Input: dimensioned drawing with shaded views. Units: mm. Origin: part minimum x, y, z. Round coordinates to 2 decimals unless told otherwise and drop trailing zeros. Loops run counter-clockwise (first coordinate to the right, second up) from the corner with the lowest first, then second, coordinate; pieces in that order, holes last. Notation, with made-up numbers: M -1,84 L 38,84 A17 ccw 38,95 Z; hole C 56,4.25 d2. An arc over 180 degrees is marked long. Return JSON: item names as keys, results as strings.
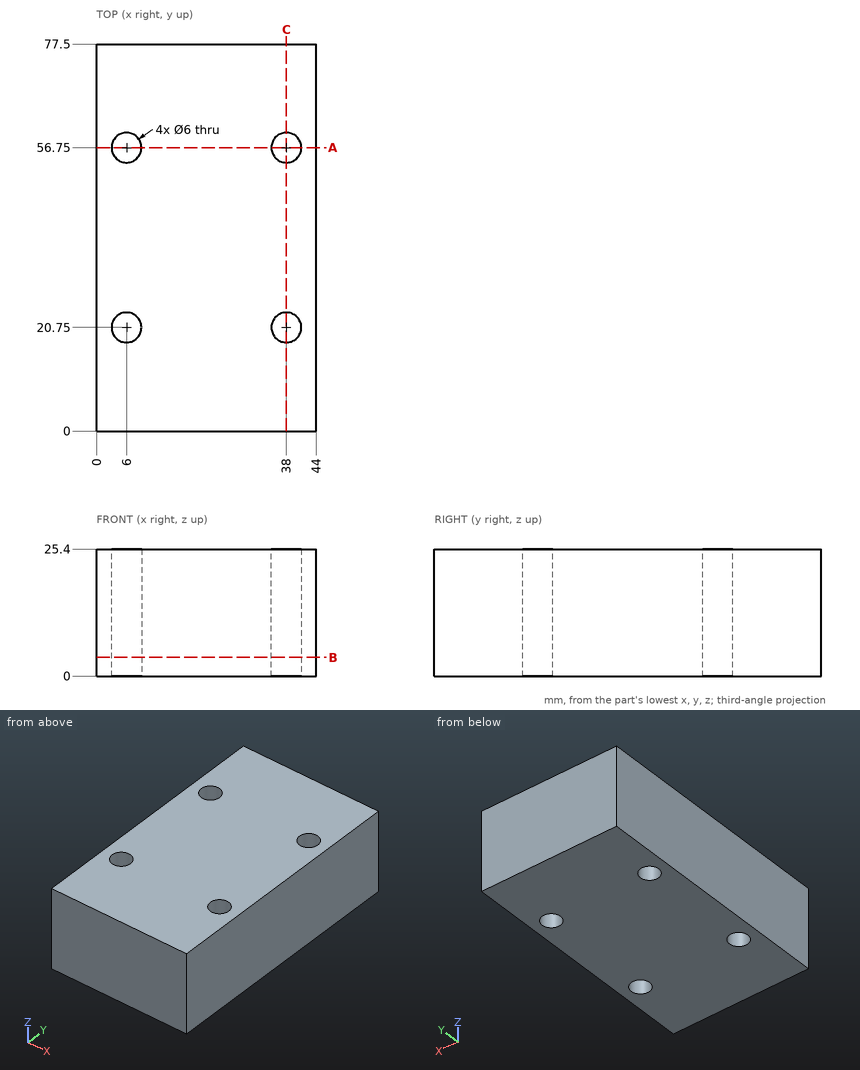
Q1. Section query A-A (y = 56.75). Output: boundary loops of the cut face in (x, z).
Determined:
{"outline": "M 0,0 L 3,0 L 3,25.4 L 0,25.4 Z; M 9,0 L 35,0 L 35,25.4 L 9,25.4 Z; M 41,0 L 44,0 L 44,25.4 L 41,25.4 Z"}
Q2. Section query C-C (x = 38). Output: boundary loops of the cut face in (y, z).
Determined:
{"outline": "M 0,0 L 17.75,0 L 17.75,25.4 L 0,25.4 Z; M 23.75,0 L 53.75,0 L 53.75,25.4 L 23.75,25.4 Z; M 59.75,0 L 77.5,0 L 77.5,25.4 L 59.75,25.4 Z"}
Q3. Section query B-B (z = 3.75). Output: boundary loops of the cut face in (x, y), plus the area to 3 significant figures.
Determined:
{"outline": "M 0,0 L 44,0 L 44,77.5 L 0,77.5 Z; hole C 6,20.75 d6; hole C 6,56.75 d6; hole C 38,20.75 d6; hole C 38,56.75 d6", "area": "3,300 mm^2"}
Q4. Material intervals for L1, parallel to Y at x = 38, z = 18.5; L2, parallel to Y at x = 3.5, z = 9.75, sorted ascending.
Determined:
{"L1": "y = 0 to 17.75, 23.75 to 53.75, 59.75 to 77.5", "L2": "y = 0 to 19.09, 22.41 to 55.09, 58.41 to 77.5"}
